Design review of the part shown in the three views and the two pictorial views. Dimensions are in mm from the part's minimum x, y and z. Round coordinates to 2 decimals unless told otherwise and drop trailing zeros. Write each loop counter-clockwise with the first axis right and the second up, starting at its lowest first coordinate (ties: lowest second). Pieces come first, ordered by that corner, then holes. Notation, with made-up numbers: (54.5, 64.5) - (75.5, 64.5) arc R25 ccw to (75.5, 76.5) - close; hole circle Ø7 at (66.25, 75). An arc over 180 degrees is marked (long way). Use one line per item in the form item = value.
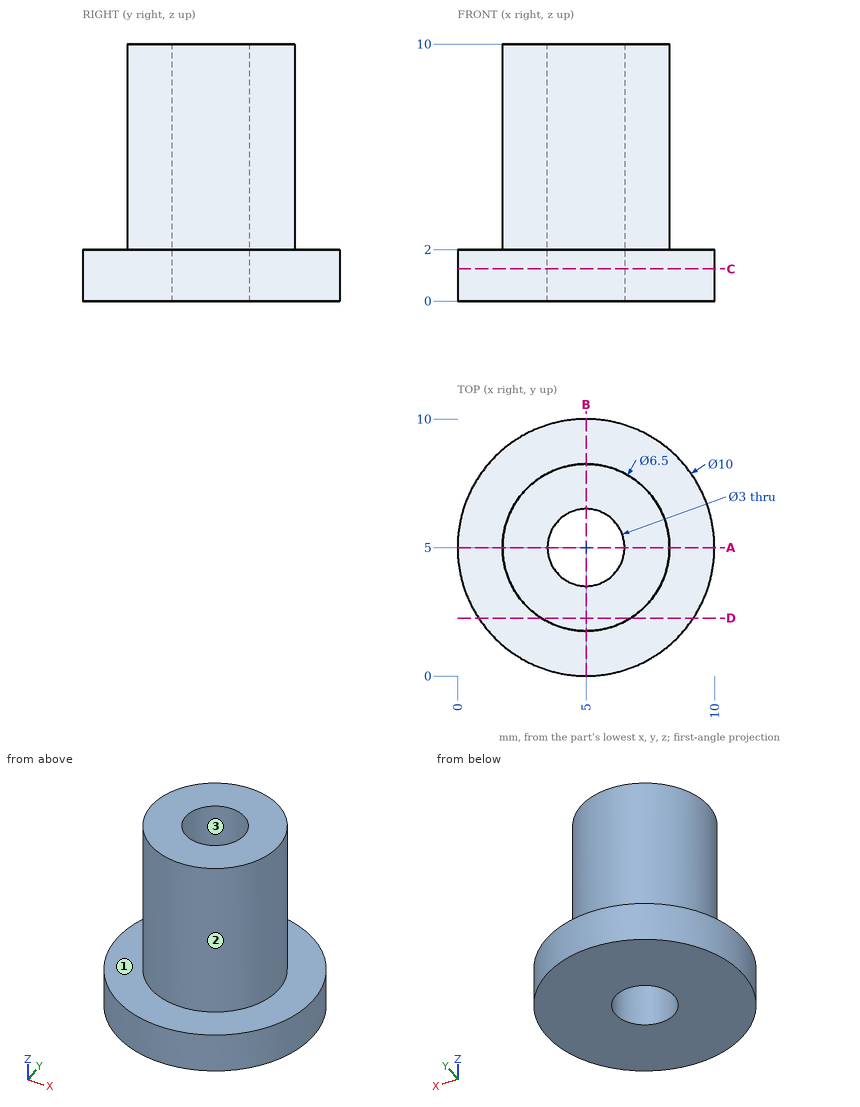
(1) Add section A-A on y = 5. Write out the cut boundary in (x, z), then the cut area to 3 significant figures.
Geometry results:
outline = (0, 0) - (3.5, 0) - (3.5, 10) - (1.75, 10) - (1.75, 2) - (0, 2) - close; (6.5, 0) - (10, 0) - (10, 2) - (8.25, 2) - (8.25, 10) - (6.5, 10) - close
area = 42.0 mm2
(2) Add section D-D on y = 2.25. Write out the cut boundary in (x, z).
Geometry results:
outline = (0.82, 0) - (9.18, 0) - (9.18, 2) - (6.73, 2) - (6.73, 10) - (3.27, 10) - (3.27, 2) - (0.82, 2) - close
(3) The part is to be moulded in two halves that separate along Y. For the marked faces 1, 2 and 3, say which applies: +Y half, -Y half, draft (parallel to the pull), parting line (faces both ways), or undercut.
Geometry results:
face_1 = draft
face_2 = parting line
face_3 = undercut
(4) To check wall thickness, follow L1, parallel to Y at x = 5, z = 2.75; L2, parallel to Z at x = 3.25, y = 9.25; L3, parallel to Y at x = 5.5, z = 9. State the ranges of each line that lie inside material, in increasing order.
Geometry results:
L1 = 1.75 to 3.5, 6.5 to 8.25
L2 = 0 to 2
L3 = 1.79 to 3.59, 6.41 to 8.21
(5) Insertion check: P1, Ø2, axis at y = 1, z = 5.5, coming from the +X side; P2, Ø1, axis at x = 4.5, y = 1, coming from the +Z side; P3, Ø5, axis at y = 7.5, z = 3, coming from the +X side. Each pin has a flat end and moves straight along its axis. Give the tip position at first contact, or say it passes through.
Geometry results:
P1 = 6.25
P2 = 2
P3 = 10
(6) Add section C-C on z = 1.25. Write out the cut boundary in (x, y).
Geometry results:
outline = circle Ø10 at (5, 5); hole circle Ø3 at (5, 5)
